Model file for the job. Use its own axes, mm. A direction names the side the tool comes from. Give positions to 0.01 mm unless a question says otherwise; leave off trailing zeros. Write each loop counter-clockwise with the first axis right and the second up, starting at its lowest first coordinate (ties: lowest second). Pieces come first, ordered by that corner, then holes. Notation, with made-up numbers: M 36.25,36.5 L 73.25,36.5 A20 cw 73.25,71.5 Z; hole C 0.5,16 d8. An arc over 180 degrees is marked long. Answer as a JSON object with one key per item and string values. Group by question number.
```python
from build123d import *

# Parameters (mm, degrees)
SKETCH1_W           = 2.7
SKETCH1_H           = 29.7
SKETCH1_W_2         = 2.8
SKETCH1_H_2         = 29.8
SKETCH1_W_3         = 2.9
SKETCH1_H_3         = 29.9
SKETCH1_W_4         = 3
SKETCH1_H_4         = 30
SKETCH1_W_5         = 3.1
SKETCH1_H_5         = 30.1
SKETCH1_W_6         = 3.2
SKETCH1_H_6         = 30.2
SKETCH1_W_7         = 3.3
SKETCH1_H_7         = 30.3
SKETCH1_W_8         = 2.6
SKETCH1_W_9         = 3.4
SKETCH1_H_8         = 30.4
BOSS_EXTRUDE1_DEPTH = 3


with BuildPart() as part:
    # Sketch1 → Boss-Extrude1 (new body)
    with BuildSketch(Plane(origin=(0, 0, 0), x_dir=(1, 0, 0), z_dir=(0, 1, 0))):
        with BuildLine():
            Line((50.7, -23.1), (-34.3, -23.1))
            ThreePointArc((-34.3, -23.1), (-37.835533906, -21.635533906), (-39.3, -18.1))
            Line((-39.3, -18.1), (-39.3, 25))
            ThreePointArc((-39.3, 25), (-37.835533906, 28.535533906), (-34.3, 30))
            Line((-34.3, 30), (50.7, 30))
            ThreePointArc((50.7, 30), (54.235533906, 28.535533906), (55.7, 25))
            Line((55.7, 25), (55.7, -18.1))
            ThreePointArc((55.7, -18.1), (54.235533906, -21.635533906), (50.7, -23.1))
        make_face()
        Polygon((1, 21), (3, 21), (3, 23), (1, 23), (1, 25), (-1, 25), (-1, 23), (-3, 23), (-3, 21), (-1, 21), (-1, 19), (1, 19), align=None, mode=Mode.SUBTRACT)
        with Locations((-24, 0)):
            Rectangle(SKETCH1_W, SKETCH1_H, mode=Mode.SUBTRACT)
        with Locations((-17, 0)):
            Rectangle(SKETCH1_W_2, SKETCH1_H_2, mode=Mode.SUBTRACT)
        with Locations((-9, 0)):
            Rectangle(SKETCH1_W_3, SKETCH1_H_3, mode=Mode.SUBTRACT)
        Rectangle(SKETCH1_W_4, SKETCH1_H_4, mode=Mode.SUBTRACT)
        with Locations((10, 0)):
            Rectangle(SKETCH1_W_5, SKETCH1_H_5, mode=Mode.SUBTRACT)
        with Locations((21, 0)):
            Rectangle(SKETCH1_W_6, SKETCH1_H_6, mode=Mode.SUBTRACT)
        with Locations((33, 0)):
            Rectangle(SKETCH1_W_7, SKETCH1_H_7, mode=Mode.SUBTRACT)
        with Locations((-30, 0)):
            Rectangle(SKETCH1_W_8, SKETCH1_H_2, mode=Mode.SUBTRACT)
        with Locations((46, 0)):
            Rectangle(SKETCH1_W_9, SKETCH1_H_8, mode=Mode.SUBTRACT)
        Polygon((16, 23), (16, 25), (19.909676119, 22), (16, 19), (16, 21), (8, 21), (8, 23), align=None, mode=Mode.SUBTRACT)
    extrude(amount=BOSS_EXTRUDE1_DEPTH)


solid = part.part
```
Q1. Slice it at B-B, the plane z = -24. Write the cut outline in (x, y).
Q2. Wall check: L1, parallel to Z at x = 22.5, y = 1.55; L2, parallel to Z at x = 46, y = 1; L3, parallel to X at y = 0.35, z = -24.5. Give the ranges that are in metal, low to high.
Q3. Two-plate mould, pull along Z, no slides. Class faces 1 (the flat face through (55.7, 1, -4)), 2 (the flat face through (-10.45, 1, 0)), 3 (the flat face through (8, 1, -30)): +Z half, -Z half, draft (parallel to the pull), parting line (faces both ways), or undercut.
Q4. 3-axis set-ups, long thin cutter, end or side, ignore diameter. For faces 4 (the cylindrical face through (-37.8, 1.48, 21.67)), 5 (the flat face through (-17, 1, 14.9)): which of +Z, -Z, +X, -X, +Y, -Y reach the whole face in a straight line?
Q5. Drop a flat-ended pin along its axis: P1, Ø2, axis at x = 10, z = -21, coming from the -Y side. Give the stop position or say it passes through.
Q6. Slice it at A-A, the plane x = 46. Write the cut outline in (y, z).
Q7. Slice it at C-C, the plane y = 1.6. Count the separate pieces of the cut face and the enclosed holes in it, then the cut area to 3 significant figures.
Solved:
{
 "1": {"outline": "M -39.3,0 L -1,0 L -1,3 L -39.3,3 Z; M 1,0 L 16,0 L 16,3 L 1,3 Z; M 17.3,0 L 55.7,0 L 55.7,3 L 17.3,3 Z"},
 "2": {"L1": "z = -30 to -15.1, 15.1 to 23.1", "L2": "z = -30 to -15.2, 15.2 to 23.1", "L3": "x = -39.3 to -1, 1 to 16, 16.65 to 55.7"},
 "3": {"face 1": "draft", "face 2": "undercut", "face 3": "-Z half"},
 "4": {"face 4": "+Z, -X, +Y, -Y", "face 5": "+Y, -Y"},
 "5": {"P1": "stops at y = 0"},
 "6": {"outline": "M 0,-30 L 3,-30 L 3,-15.2 L 0,-15.2 Z; M 0,15.2 L 3,15.2 L 3,23.1 L 0,23.1 Z"},
 "7": {"separate pieces": "1", "enclosed holes": "11", "area": "4,160 mm²"}
}
